Could you check a few things on this model? Use its own coordinates, in mm. Face numbers are marked on the shaded views. A direction names the side the tool comes from. Round coordinates to 2 decimals unless told otherwise and drop trailing zeros. Loops run counter-clockwise (first coordinate to the right, second up) from the corner with the lowest first, then second, coordinate; pieces in that order, holes last. Notation, with made-up numbers: (49, 27) -> (101, 27) arc R14 cw to (101, 51) -> close; hole circle Ø10 at (10.25, -26). An arc over 180 degrees is marked (long way). One line per item, written item: value.
```python
from build123d import *

# Parameters (mm, degrees)
F1_DEPTH = 54
F3_D     = 38
F5_D     = 6.3
F5_DEPTH = 12
F5_TIP   = 1.8927109499


# Not quite as in the source:
# - a feature names something its author has since deleted; it is built from what else it names


with BuildPart() as f1:
    # F0 (on Front) → F1 (new body)
    with BuildSketch(Plane.XZ):
        Polygon((28.0907023698, -33.5), (33.5, -33.5), (33.5, -25.5690795523), (31.4847062311, -23.5432559017), (26.8295921046, -32.2290576438), align=None)
        Polygon((-25.1683651974, -33.5), (28.0907023698, -33.5), (26.8295921046, -32.2290576438), (0.4087149623, -5.6021933843), (-23.8942493722, -32.1102777692), align=None)
        Polygon((31.4847062311, -23.5432559017), (33.5, -25.5690795523), (33.5, 30.4916165769), (32.4673100421, 29.3652258959), (6.7529691073, 1.3177042019), align=None)
        Polygon((-33.5, -33.5), (-25.1683651974, -33.5), (-23.8942493722, -32.1102777692), (-30.7295821389, -25.7524549578), (-33.5, -28.7309475243), align=None)
        Polygon((32.4673100421, 29.3652258959), (33.5, 30.4916165769), (33.5, 33.5), (24.3835517234, 33.5), (22.7440218852, 31.7373318104), align=None)
        Polygon((-33.5, 28.5708867013), (-33.5, -28.7309475243), (-30.7295821389, -25.7524549578), (-5.9894273378, 0.8458312449), (-30.3316890574, 25.3778744124), align=None)
        Polygon((22.7440218852, 31.7373318104), (24.3835517234, 33.5), (-25.2620486716, 33.5), (-23.714253223, 31.9441173419), (0.3945803139, 7.7093154877), align=None)
        Polygon((-33.5, 33.5), (-33.5, 28.5708867013), (-30.3316890574, 25.3778744124), (-23.714253223, 31.9441173419), (-25.2620486716, 33.5), align=None)
    extrude(amount=-F1_DEPTH)

    # F3 (through all)
    with Locations(Plane.YZ.offset(33.5)):
        with Locations((28.3605195582, -6.5)):
            Hole(F3_D / 2)

    # F5
    with Locations(Plane.XY.offset(33.5)):
        with Locations((0, 49.4885705411)):
            Hole(F5_D / 2, depth=F5_DEPTH)
            with Locations((0, 0, -(F5_DEPTH + F5_TIP / 2))):  # 118° drill point
                Cone(0, F5_D / 2, F5_TIP, mode=Mode.SUBTRACT)


solid = f1.part
```
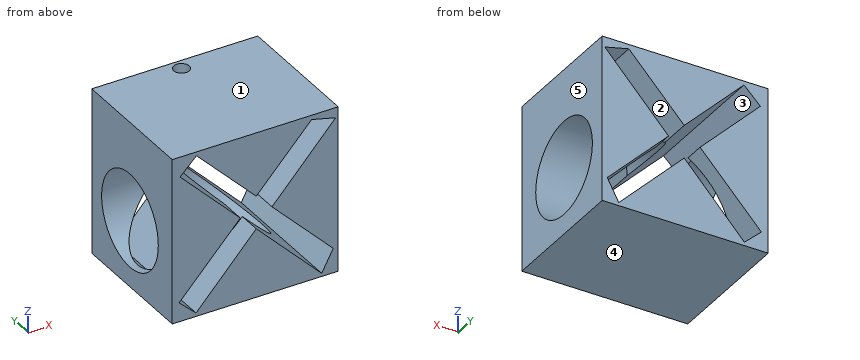
Item 1: If we section it at C-C on z = -4.5: List the corners of the cut face in (x, y) for me.
Output:
outline: (-33.5, 0) -> (-10.96, 0) -> (-10.96, 9.47) -> (-33.5, 9.47) -> close; (-33.5, 47.25) -> (-10.96, 47.25) -> (-10.96, 54) -> (-33.5, 54) -> close; (12.54, 0) -> (33.5, 0) -> (33.5, 9.47) -> (12.54, 9.47) -> close; (12.54, 47.25) -> (33.5, 47.25) -> (33.5, 54) -> (12.54, 54) -> close
Item 2: If we section it at D-D on x = 9: List the corners of the cut face in (y, z) for me.
Output:
outline: (0, -33.5) -> (54, -33.5) -> (54, -14.26) -> (45.7, -14.26) arc R19 cw to (11.02, -14.26) -> (0, -14.26) -> close; (0, -0.94) -> (10.19, -0.94) arc R19 cw to (12.37, 3.77) -> (0, 3.77) -> close; (0, 16.96) -> (54, 16.96) -> (54, 33.5) -> (0, 33.5) -> close; (44.35, 3.77) arc R19 cw to (46.53, -0.94) -> (54, -0.94) -> (54, 3.77) -> close
Item 3: For the marked faces 1 and 2, which set-ups out of +Z, -Z, +X, -X, +Y, -Y let a thin tool reach every point of the face, with its end or its side?
Output:
face 1: +Z, +X, -X, +Y, -Y
face 2: +Y, -Y
Item 4: If we section it at A-A on z = 28: List the corners of the cut face in (x, y) for me, plus the area to 3 significant figures.
Output:
outline: (-33.5, 0) -> (-27.69, 0) -> (-27.69, 54) -> (-33.5, 54) -> close; (-19.79, 0) -> (19.27, 0) -> (19.27, 54) -> (-19.79, 54) -> close; (31.22, 0) -> (33.5, 0) -> (33.5, 54) -> (31.22, 54) -> close; hole circle Ø6.3 at (0, 49.49)
area: 2,520 mm²
Item 5: If we mould it in two halves opening along Z, with no side actions, what happens to the marked faces 3, 4 and 5? For each: released by +Z, released by -Z, zero draft, split by the parting line, or undercut.
Output:
face 3: undercut
face 4: released by -Z
face 5: zero draft
Item 6: Will this pin go through, and if not, where does the flat tip stop? pin 1 Ø3 at (x, z) = (21.5, 16.5) entering from -Y.
Output:
pin 1: stops at y = 0
Item 7: I need wall thicknesses on line 1 (Y direction, x = 28, z = -6.5); line 2 (X direction, y = 6, z = -6); line 3 (X direction, y = 34, z = -25). Which ranges of each line are inside material? Lowest first, please. Write a range as from..to.
Output:
line 1: y = 0..9.36, 47.36..54
line 2: x = -33.5..-12.36, 0.04..0.8, 14.03..33.5
line 3: x = -33.5..-30.03, -17.38..19.66, 30.7..33.5
Item 8: If we section it at B-B on y = 32.5: List the corners of the cut face in (x, z) for me, plus the area to 3 significant figures.
Output:
outline: (-33.5, -33.5) -> (33.5, -33.5) -> (33.5, -25.04) -> (30.68, -25.04) -> (26.83, -32.23) -> (19.7, -25.04) -> (-17.42, -25.04) -> (-23.89, -32.11) -> (-30.73, -25.75) -> (-30.07, -25.04) -> (-33.5, -25.04) -> close; (-33.5, 12.04) -> (-17.1, 12.04) -> (-30.33, 25.38) -> (-23.71, 31.94) -> (-3.92, 12.04) -> (4.43, 12.04) -> (22.74, 31.74) -> (32.47, 29.37) -> (16.59, 12.04) -> (33.5, 12.04) -> (33.5, 33.5) -> (-33.5, 33.5) -> close
area: 1,470 mm²
